The model under review builds one solid part; all positions refer to its coordinate system, in mm. Face numbers are marked on the shaded views. A direction names the side the tool comes from. Coordinates: 2 decimals unless noted, no trailing zeros. Write each loop counter-clockwise with the first axis right and the second up, starting at its lowest first coordinate (ties: lowest second). Pieces come first, ordered by that corner, then holes. Notation, with made-up numbers: (62.5, 85) -> (95.5, 85) arc R30 ccw to (95.5, 123) -> close; hole circle Ø5 at (29, 56). An arc over 180 degrees is marked (long way). Put each result on its own line as item: value. Start each with the question number.
from build123d import *

# Parameters (mm, degrees)
ESQUISSE1_R             = 24.5
ESQUISSE1_R_2           = 18.5
BOSS_EXTRU_1_DEPTH      = 20
ENL_V_MAT_EXTRU_1_DEPTH = 21
BOSS_EXTRU_2_DEPTH      = 20
ESQUISSE4_R             = 21.5
BOSS_EXTRU_3_DEPTH      = 4.5
ENL_V_MAT_EXTRU_2_REACH = 6.5
ESQUISSE5_R             = 2


with BuildPart() as part:
    # Esquisse1 → Boss.-Extru.1 (new body)
    with BuildSketch(Plane(origin=(0, 0, 0), x_dir=(1, 0, 0), z_dir=(0, 1, 0))):
        Circle(ESQUISSE1_R)
        Circle(ESQUISSE1_R_2, mode=Mode.SUBTRACT)
    extrude(amount=BOSS_EXTRU_1_DEPTH)

    # Esquisse2 → Enlèv. mat.-Extru.1 (cut, through all)
    with BuildSketch(Plane(origin=(0, 20, 0), x_dir=(1, 0, 0), z_dir=(0, 1, 0))):
        with BuildLine():
            ThreePointArc((-12.25, 21.217622393), (-21.217622393, 12.25), (-24.5, 0))
            ThreePointArc((-24.5, 0), (-23, -1.5), (-21.5, 0))
            ThreePointArc((-21.5, 0), (-18.619546181, 10.75), (-10.75, 18.619546181))
            ThreePointArc((-10.75, 18.619546181), (-10.200961894, 20.668584287), (-12.25, 21.217622393))
        make_face()
        with BuildLine():
            ThreePointArc((24.5, 0), (21.217622393, 12.25), (12.25, 21.217622393))
            ThreePointArc((12.25, 21.217622393), (10.200961894, 20.668584287), (10.75, 18.619546181))
            ThreePointArc((10.75, 18.619546181), (18.619546181, 10.75), (21.5, 0))
            ThreePointArc((21.5, 0), (23, -1.5), (24.5, 0))
        make_face()
        with BuildLine():
            ThreePointArc((-12.25, -21.217622393), (0, -24.5), (12.25, -21.217622393))
            ThreePointArc((12.25, -21.217622393), (12.799038106, -19.168584287), (10.75, -18.619546181))
            ThreePointArc((10.75, -18.619546181), (0, -21.5), (-10.75, -18.619546181))
            ThreePointArc((-10.75, -18.619546181), (-12.799038106, -19.168584287), (-12.25, -21.217622393))
        make_face()
    extrude(amount=-ENL_V_MAT_EXTRU_1_DEPTH, mode=Mode.SUBTRACT)

    # Esquisse3 → Boss.-Extru.2 (add)
    with BuildSketch(Plane(origin=(0, 20, 0), x_dir=(1, 0, 0), z_dir=(0, 1, 0))):
        with BuildLine():
            ThreePointArc((19.445436483, 19.445436483), (0, 27.5), (-19.445436483, 19.445436483))
            ThreePointArc((-19.445436483, 19.445436483), (-19.445436483, 17.324116139), (-17.324116139, 17.324116139))
            ThreePointArc((-17.324116139, 17.324116139), (0, 24.5), (17.324116139, 17.324116139))
            ThreePointArc((17.324116139, 17.324116139), (19.445436483, 17.324116139), (19.445436483, 19.445436483))
        make_face()
        with BuildLine():
            ThreePointArc((7.11752374, -26.562960223), (23.815698604, -13.75), (26.562960223, 7.11752374))
            ThreePointArc((26.562960223, 7.11752374), (24.725842916, 8.178183912), (23.665182744, 6.341066605))
            ThreePointArc((23.665182744, 6.341066605), (21.217622393, -12.25), (6.341066605, -23.665182744))
            ThreePointArc((6.341066605, -23.665182744), (5.280406433, -25.502300051), (7.11752374, -26.562960223))
        make_face()
        with BuildLine():
            ThreePointArc((-26.562960223, 7.11752374), (-23.815698604, -13.75), (-7.11752374, -26.562960223))
            ThreePointArc((-7.11752374, -26.562960223), (-5.280406433, -25.502300051), (-6.341066605, -23.665182744))
            ThreePointArc((-6.341066605, -23.665182744), (-21.217622393, -12.25), (-23.665182744, 6.341066605))
            ThreePointArc((-23.665182744, 6.341066605), (-24.725842916, 8.178183912), (-26.562960223, 7.11752374))
        make_face()
    extrude(amount=-BOSS_EXTRU_2_DEPTH)

    # Esquisse4 → Boss.-Extru.3 (add)
    with BuildSketch(Plane.XZ):
        Circle(ESQUISSE4_R)
    extrude(amount=-BOSS_EXTRU_3_DEPTH)

    # Esquisse5 → Enlèv. mat.-Extru.2 (cut, up to next)
    with BuildSketch(Plane(origin=(0, 4.5, 0), x_dir=(1, 0, 0), z_dir=(0, 1, 0)), mode=Mode.PRIVATE) as enl_v_mat_extru_2_sk1:
        with Locations((0, 13)):
            Circle(ESQUISSE5_R)
    enl_v_mat_extru_2_tool1 = extrude(enl_v_mat_extru_2_sk1.sketch, amount=-ENL_V_MAT_EXTRU_2_REACH, mode=Mode.PRIVATE) & part.part
    add(enl_v_mat_extru_2_tool1.solids().sort_by_distance((0, 4.5, -13))[0], mode=Mode.SUBTRACT)
    # Esquisse5 → Enlèv. mat.-Extru.2 (cut, up to next)
    with BuildSketch(Plane(origin=(0, 4.5, 0), x_dir=(1, 0, 0), z_dir=(0, 1, 0)), mode=Mode.PRIVATE) as enl_v_mat_extru_2_sk2:
        with Locations((11.258330249, -6.5)):
            Circle(ESQUISSE5_R)
    enl_v_mat_extru_2_tool2 = extrude(enl_v_mat_extru_2_sk2.sketch, amount=-ENL_V_MAT_EXTRU_2_REACH, mode=Mode.PRIVATE) & part.part
    add(enl_v_mat_extru_2_tool2.solids().sort_by_distance((11.25833, 4.5, 6.5))[0], mode=Mode.SUBTRACT)
    # Esquisse5 → Enlèv. mat.-Extru.2 (cut, up to next)
    with BuildSketch(Plane(origin=(0, 4.5, 0), x_dir=(1, 0, 0), z_dir=(0, 1, 0)), mode=Mode.PRIVATE) as enl_v_mat_extru_2_sk3:
        with Locations((-11.258330249, -6.5)):
            Circle(ESQUISSE5_R)
    enl_v_mat_extru_2_tool3 = extrude(enl_v_mat_extru_2_sk3.sketch, amount=-ENL_V_MAT_EXTRU_2_REACH, mode=Mode.PRIVATE) & part.part
    add(enl_v_mat_extru_2_tool3.solids().sort_by_distance((-11.25833, 4.5, 6.5))[0], mode=Mode.SUBTRACT)


solid = part.part
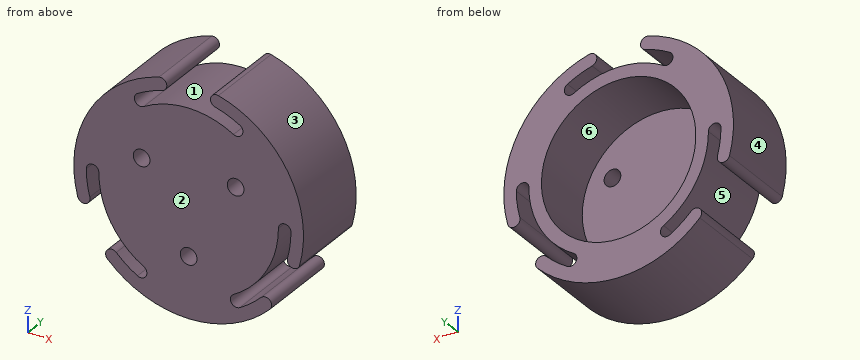
1. Consider section D-D on z = -13. State the section outline as (x, y) points.
2. Tool access review of the marked faces 4, 5 and 6: name each direction out of +Z, -Z, +X, -X, +Y, -Y from which nothing blocks a thin tool from reaching the whole face with its end or side.
3. Consider section A-A on y = 5.75. State the section outline as (x, z) points, then the cut area to 3 significant figures.
4. Insertion check: P1, Ø11, axis at x = 3.5, z = 1.5, coming from the +Y side; P2, Ø6, axis at y = 11.5, z = 6.5, coming from the -X side; P3, Ø6, axis at y = 6.5, z = 12, coming from the -X side; P4, Ø3.5, axis at x = 11.26, z = 6.5, coming from the -Y side. Each pin has a flat end and moves straight along its axis. Give the tip position at first contact, or say it passes through.
5. The part is to be moulded in two halves that separate along X. For the marked faces 1, 2 and 3, say which applies: released by +X, released by -X, zero draft, split by the parting line, or undercut.
6. Wall thickness on line 1 (Z direction, x = -8, y = 7); line 2 (Z direction, x = 0, y = 2.1); line 3 (X direction, y = 2.45, z = 6.5): over which ranges is each line inside the solid? List them lowest first. Write a range as from..to.
7. Consider section C-C on x = -16. State the section outline as (y, z) points, then the cut area to 3 significant figures.
8. Consider section B-B on x = 11.5. State the section outline as (y, z) points, then the cut area to 3 significant figures.
Output values:
1. outline: (-17.12, 0) -> (-2, 0) -> (-2, 4.5) -> (-13.16, 4.5) -> (-13.16, 20) -> (-17.12, 20) -> close; (2, 0) -> (17.12, 0) -> (17.12, 20) -> (13.16, 20) -> (13.16, 4.5) -> (2, 4.5) -> close
2. face 4: -X, +Y, -Y
2. face 5: +Y, -Y
2. face 6: +Y
3. outline: (-26.56, -7.12) arc R1.5 ccw to (-23.67, -6.34) arc R24.5 cw to (-24.5, 0) arc R1.5 cw to (-21.5, 0) arc R21.5 ccw to (-10.75, -18.62) arc R1.5 cw to (-12.25, -21.22) arc R24.5 cw to (-17.32, -17.32) arc R1.5 ccw to (-19.45, -19.45) arc R27.5 ccw to (19.45, -19.45) arc R1.5 ccw to (17.32, -17.32) arc R24.5 cw to (12.25, -21.22) arc R1.5 cw to (10.75, -18.62) arc R21.5 ccw to (21.5, 0) arc R1.5 cw to (24.5, 0) arc R24.5 cw to (23.67, -6.34) arc R1.5 ccw to (26.56, -7.12) arc R27.5 ccw to (7.12, 26.56) arc R1.5 ccw to (6.34, 23.67) arc R24.5 cw to (12.25, 21.22) arc R1.5 cw to (10.75, 18.62) arc R21.5 ccw to (-10.75, 18.62) arc R1.5 cw to (-12.25, 21.22) arc R24.5 cw to (-6.34, 23.67) arc R1.5 ccw to (-7.12, 26.56) arc R27.5 ccw to start; hole circle Ø37 at (0, 0)
3. area: 961 mm^2
4. P1: stops at y = 4.5
4. P2: stops at x = -27.28
4. P3: stops at x = -25.99
4. P4: passes through
5. face 1: undercut
5. face 2: zero draft
5. face 3: released by +X
6. line 1: z = -26.31..-16.68, 16.68..19.96, 23.16..26.31
6. line 2: z = -27.5..-15, -11..21.5
6. line 3: x = -26.72..-13.26, -9.26..9.26, 13.26..26.72
7. outline: (0, -22.37) -> (20, -22.37) -> (20, -18.55) -> (0, -18.55) -> close; (0, -14.36) -> (20, -14.36) -> (20, -9.29) -> (4.5, -9.29) -> (4.5, 9.29) -> (20, 9.29) -> (20, 22.37) -> (0, 22.37) -> close
7. area: 523 mm^2
8. outline: (0, -24.98) -> (20, -24.98) -> (20, -21.42) -> (0, -21.42) -> close; (0, -18.17) -> (20, -18.17) -> (20, -14.49) -> (4.5, -14.49) -> (4.5, 4.51) -> (0, 4.51) -> close; (0, 8.49) -> (4.5, 8.49) -> (4.5, 14.49) -> (20, 14.49) -> (20, 18.42) -> (0, 18.42) -> close; (0, 21.63) -> (20, 21.63) -> (20, 24.98) -> (0, 24.98) -> close
8. area: 403 mm^2
